Here's how the part is built. I have some questions about the finished solid (model axes, mm). Face numbers are marked on the shaded views. Give positions to 0.01 mm unless a question says otherwise; leave off trailing zeros. Write each loop counter-clockwise with the first axis right and the second up, starting at its lowest first coordinate (ties: lowest second). Pieces come first, ordered by that corner, then holes. Notation, with made-up numbers: (-29.5, -11.5) -> (13.5, -11.5) arc R11 ccw to (13.5, -6.5) -> close; hole circle Ø10 at (37.25, -24). An arc over 180 degrees is marked (long way). Use one line per item in the form item = value.
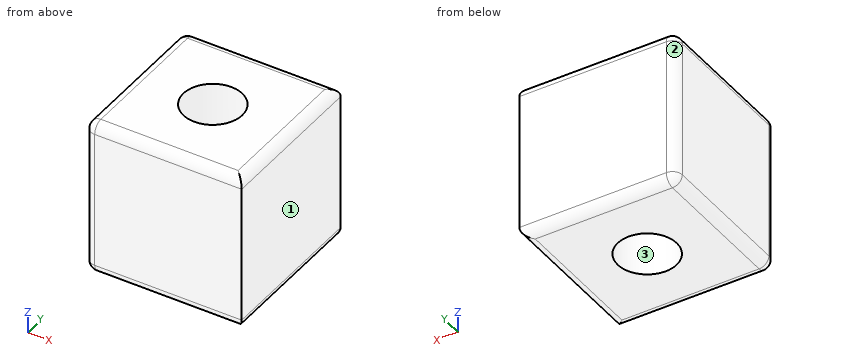
```python
from build123d import *

# Parameters (mm, degrees)
F0_W     = 80
F0_H     = 80
F1_DEPTH = 40
F2_R     = 5
F3_R     = 15
F4_DEPTH = 80.001


with BuildPart() as f1:
    # F0 (on Top) → F1 (new body, symmetric)
    with BuildSketch(Plane.XY):
        Rectangle(F0_W, F0_H)
    extrude(amount=F1_DEPTH, both=True)

    # F2
    f2_edges = [f1.edges().sort_by_distance(p)[0] for p in [
        (40, 0, 40),
        (0, 40, 40),
        (-40, 0, 40),
        (0, -40, 40),
        (-40, 40, 0),
        (-40, 0, -40),
        (-40, -40, 0),
        (0, 40, -40),
        (0, -40, -40),
        (40, 0, -40),
    ]]
    fillet(f2_edges, radius=F2_R)

    # F3 (on face) → F4 (cut, through all)
    with BuildSketch(Plane.XY.offset(40)):
        Circle(F3_R)
    extrude(amount=-F4_DEPTH, mode=Mode.SUBTRACT)


solid = f1.part
```
Q1. I want a section at C-C, the plane z = -31.5. Write out the boundary of the cut face in (x, y), and give its area (3 significant figures).
Result set:
outline = (-40, -35) arc R5 ccw to (-35, -40) -> (40, -40) -> (40, 40) -> (-35, 40) arc R5 ccw to (-40, 35) -> close; hole circle Ø30 at (0, 0)
area = 5,680 mm2
Q2. If I drill on line 1 along Y through (x, z) = (0, 13); line 2 along X through (y, z) = (4, -17); line 3 along X through (y, z) = (-11.5, 33), over which ranges is the centre line in solid material (lowest first)? Write a range as from..to.
Result set:
line_1 = -40..-15, 15..40
line_2 = -40..-14.46, 14.46..40
line_3 = -40..-9.63, 9.63..40
Q3. If we mould it in two halves opening along X, with no side actions, what happens to the marked faces 1, 2 and 3? For each: +X half, -X half, draft (parallel to the pull), parting line (faces both ways), or undercut.
Result set:
face_1 = +X half
face_2 = -X half
face_3 = undercut
Q4. I want a section at A-A, the plane x = 0. Write out the boundary of the cut face in (y, z).
Result set:
outline = (-40, -35) arc R5 ccw to (-35, -40) -> (-15, -40) -> (-15, 40) -> (-35, 40) arc R5 ccw to (-40, 35) -> close; (15, -40) -> (35, -40) arc R5 ccw to (40, -35) -> (40, 35) arc R5 ccw to (35, 40) -> (15, 40) -> close
